from build123d import *

# Parameters (mm, degrees)
SKETCH18_R           = 31.5
BOSS_EXTRUDE13_DEPTH = 8
SKETCH19_R           = 2
BOSS_EXTRUDE14_DEPTH = 2


with BuildPart() as part:
    # Sketch18 → Boss-Extrude13 (new body)
    with BuildSketch(Plane(origin=(0, 0, 0), x_dir=(1, 0, 0), z_dir=(0, 1, 0))):
        with BuildLine():
            Line((-39.5, 0), (-39.5, 42.5))
            Line((-39.5, 42.5), (39.5, 42.5))
            Line((39.5, 42.5), (39.5, 0))
            ThreePointArc((39.5, 0), (0, -39.5), (-39.5, 0))
        make_face()
        Circle(SKETCH18_R, mode=Mode.SUBTRACT)
    extrude(amount=BOSS_EXTRUDE13_DEPTH)

    # Sketch19 → Boss-Extrude14 (add)
    with BuildSketch(Plane.XZ):
        with Locations((-35.5, -38.5)):
            Circle(SKETCH19_R)
        with Locations((35.5, -38.5)):
            Circle(SKETCH19_R)
    extrude(amount=BOSS_EXTRUDE14_DEPTH)


solid = part.part
The model under review builds one solid part; all positions refer to its coordinate system, in mm. A direction names the side the tool comes from. Round coordinates to 2 decimals unless told otherwise and drop trailing zeros. Loops run counter-clockwise (first coordinate to the right, second up) from the corner with the lowest first, then second, coordinate; pieces in that order, holes last. Notation, with made-up numbers: (-1.75, 60.5) -> (51.25, 60.5) arc R25 ccw to (51.25, 72.5) -> close; hole circle Ø9 at (10, 13). An arc over 180 degrees is marked (long way). Return JSON: item names as keys, results as strings.
(1) For line 1 (Z direction, x = 0, y = 3.5); line 2 (Y direction, x = 35, z = -12); line 3 (Z direction, x = -18, y = 3), list the stretches that pass through material, from the lowest coordinate up.
Solved:
{"line 1": "-42.5 to -31.5, 31.5 to 39.5", "line 2": "0 to 8", "line 3": "-42.5 to -25.85, 25.85 to 35.16"}
(2) Add section A-A on x = 0. Write out the cut boundary in (y, z), plus the area to 3 significant figures.
Solved:
{"outline": "(0, -42.5) -> (8, -42.5) -> (8, -31.5) -> (0, -31.5) -> close; (0, 31.5) -> (8, 31.5) -> (8, 39.5) -> (0, 39.5) -> close", "area": "152 mm2"}
(3) Add section C-C on y = 5.75. Write out the cut boundary in (x, z).
Solved:
{"outline": "(-39.5, -42.5) -> (39.5, -42.5) -> (39.5, 0) arc R39.5 ccw to (-39.5, 0) -> close; hole circle Ø63 at (0, 0)"}
(4) For faces 1 (the flat face through (18, 8, -29)), 2 (the cylindrical face through (36.423, -0.986, -40.274)), list the 3-axis set-ups (+Z, -Z, +X, -X, +Y, -Y) from which the entire face can be reached by the end or side of a thin tool; tool diameter is ignored.
Solved:
{"face 1": "+Z, -Z, +X, -X, +Y", "face 2": "-Y"}
(5) For pin 1 (5 mm diameter, centred on y = -0.5, z = 24, fed in from +X); pin 2 (2 mm diameter, centred on y = 3, z = 5.5, fed in from +X), all flat-tipped, find the tip position at first contact; note any pin that passes through.
Solved:
{"pin 1": "x = 33.1", "pin 2": "x = 39.24"}
(6) Add section B-B on z = 10.5. Write out the cut boundary in (x, y).
Solved:
{"outline": "(-38.08, 0) -> (-29.7, 0) -> (-29.7, 8) -> (-38.08, 8) -> close; (29.7, 0) -> (38.08, 0) -> (38.08, 8) -> (29.7, 8) -> close"}
(7) Add section D-D on z = -38.5. Write out the cut boundary in (x, y).
Solved:
{"outline": "(-39.5, 0) -> (-37.5, 0) -> (-37.5, -2) -> (-33.5, -2) -> (-33.5, 0) -> (33.5, 0) -> (33.5, -2) -> (37.5, -2) -> (37.5, 0) -> (39.5, 0) -> (39.5, 8) -> (-39.5, 8) -> close"}
(8) The part is to be moulded in two halves that separate along X. For faces 3 (the cylindrical face through (-4.101, 3.944, -31.232)), 4 (the flat face through (39.5, 4, -22)), 5 (the cylindrical face through (0.87, 3.94, 39.49)), 6 (the flat face through (35, -2, -38)), say which applies: released by +X, released by -X, zero draft, split by the parting line, or undercut.
Solved:
{"face 3": "undercut", "face 4": "released by +X", "face 5": "split by the parting line", "face 6": "zero draft"}
